Read the model definition and answer for the solid it produces. Units are mm, in the model's axes. Face numbers are marked on the shaded views. A direction names the side the tool comes from. Coordinates: 2 decimals unless noted, no trailing zeros. Loops run counter-clockwise (first coordinate to the right, second up) from the corner with the lowest first, then second, coordinate; pieces in that order, holes last. Notation, with made-up numbers: M 5.5,42.5 L 61.5,42.5 A30 ccw 61.5,68.5 Z; hole C -27,78.5 d4. An arc over 180 degrees is marked long. Use one line per item in the form item = value. Start each with the question number.
1. The part is cut by section A-A (x = 14.75). Give the number of separate pieces and of enclosed holes in the cut face, plus the area to 3 significant figures.
2. For a pull along Y with two mould halves and no side action, classify the marked faces 3, 4, 5 and 6 as released by +Y, released by -Y, zero draft, split by the parting line, or undercut.
3. A tool of negligible diameter and unlimited length cuts with its end or side. For the marked faces 1 and 2, from which of +Z, -Z, +X, -X, +Y, -Y can it reach the whole face along a straight path? Write none if from no direction.
4. The part is cut by section C-C (y = -11.5). Give the vertices of the cut face in (x, z).
5. The part is cut by section B-B (z = 63). Give the vertices of the cut face in (x, y), plus the area to 3 significant figures.
6. Find the intervals of material crossed by probe 1 along Y at (x, z) = (5, -84.05); probe 2 along Y at (x, z) = (6.5, -60.5); probe 3 along Y at (x, z) = (17.25, 28), in increasing order. Write a range as [from, to].
from build123d import *

# Parameters (mm, degrees)
SKETCH4_W           = 170
SKETCH4_H           = 50
BOSS_EXTRUDE1_DEPTH = 20
CUT_EXTRUDE5_DEPTH  = 20
CUT_EXTRUDE6_DEPTH  = 20
SKETCH7_R           = 3
SKETCH7_R_2         = 2
CUT_EXTRUDE7_DEPTH  = 5
SKETCH8_R           = 3
SKETCH8_R_2         = 2
CUT_EXTRUDE8_DEPTH  = 5


with BuildPart() as part:
    # Sketch4 → Boss-Extrude1 (new body)
    with BuildSketch(Plane(origin=(0, 0, 0), x_dir=(0, 0, -1), z_dir=(1, 0, 0))):
        Rectangle(SKETCH4_W, SKETCH4_H)
    extrude(amount=BOSS_EXTRUDE1_DEPTH)

    # Sketch5 → Cut-Extrude5 (cut)
    with BuildSketch(Plane.ZY):
        Polygon((-82.5, 20), (82.5, 20), (0, 2.648640731), align=None)
        Polygon((0, -1.957690975), (82.5, -20), (-82.5, -20), align=None)
    extrude(amount=-CUT_EXTRUDE5_DEPTH, mode=Mode.SUBTRACT)

    # Sketch6 → Cut-Extrude6 (cut)
    with BuildSketch(Plane.ZY):
        Polygon((-2.994115609, 0), (-81.99270438, 17.619218778), (-81.99270438, -17.158585608), align=None)
        Polygon((2.994115609, 0), (82.148587467, 16.647729441), (82.148587467, -17.653985706), align=None)
    extrude(amount=-CUT_EXTRUDE6_DEPTH, mode=Mode.SUBTRACT)

    # Sketch7 → Cut-Extrude7 (cut)
    with BuildSketch(Plane.XY.offset(85)):
        with Locations((9.915502372, 0.478984513)):
            Circle(SKETCH7_R)
        with Locations((4.915502372, -4.521015487)):
            Circle(SKETCH7_R_2)
        with Locations((14.915502372, -4.521015487)):
            Circle(SKETCH7_R_2)
        with Locations((14.915502372, 5.478984513)):
            Circle(SKETCH7_R_2)
        with Locations((4.915502372, 5.478984513)):
            Circle(SKETCH7_R_2)
    extrude(amount=-CUT_EXTRUDE7_DEPTH, mode=Mode.SUBTRACT)

    # Sketch8 → Cut-Extrude8 (cut)
    with BuildSketch(Plane(origin=(0, 0, -85), x_dir=(-1, 0, 0), z_dir=(0, 0, -1))):
        with Locations((-10, 0)):
            Circle(SKETCH8_R)
        with Locations((-15, 5)):
            Circle(SKETCH8_R_2)
        with Locations((-5, 5)):
            Circle(SKETCH8_R_2)
        with Locations((-5, -5)):
            Circle(SKETCH8_R_2)
        with Locations((-15, -5)):
            Circle(SKETCH8_R_2)
    extrude(amount=-CUT_EXTRUDE8_DEPTH, mode=Mode.SUBTRACT)


solid = part.part
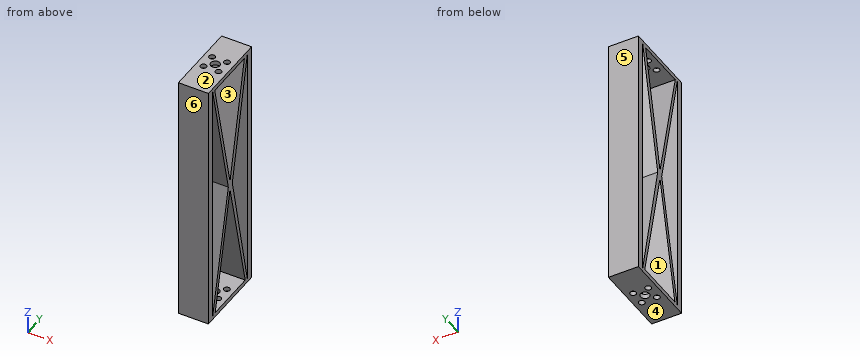
Computed values:
q1.separate_pieces = 3
q1.enclosed_holes = 2
q1.area = 2,800 mm²
q2.face_3 = undercut
q2.face_4 = zero draft
q2.face_5 = released by +Y
q2.face_6 = released by -Y
q3.face_1 = +X, -X
q3.face_2 = +Z, +X, -X, +Y, -Y
q4.outline = M 0,-85 L 20,-85 L 20,-81.99 L 0,-81.99 Z; M 0,-55.94 L 20,-55.94 L 20,-43.63 L 0,-43.63 Z; M 0,43.63 L 20,43.63 L 20,54.56 L 0,54.56 Z; M 0,82.15 L 20,82.15 L 20,85 L 0,85 Z
q5.outline = M 0,-25 L 20,-25 L 20,-20 L 0,-20 Z; M 0,-15.74 L 20,-15.74 L 20,-13.38 L 0,-13.38 Z; M 0,12.62 L 20,12.62 L 20,15.9 L 0,15.9 Z; M 0,20 L 20,20 L 20,25 L 0,25 Z
q5.area = 313 mm²
q6.probe_1 = [-25, -7], [-3, 3], [7, 25]
q6.probe_2 = [-25, -20], [-15.19, -12.49], [12.83, 15.37], [20, 25]
q6.probe_3 = [-25, -20], [-8.08, -5.58], [5.26, 8.54], [20, 25]
